Work out the finished part from the listing and answer in its coordinate system (mm). A direction names the side the tool comes from. Coordinates: 2 decimals unless noted, no trailing zeros. Order: outer loops, then holes, each group sorted by start corner. A loop starts at its lowest first (then second) coordinate and runs counter-clockwise, first axis right, second up.
1. The part is cut by section C-C, the plane y = -0.75. Give the vertices of the cut face in (x, z).
2. The part is cut by section D-D, the plane x = 0.4. Give the vertices of the cut face in (y, z).
3. Find the intervals of material crossed by probe 1 along Z at (x, y) = (-1.3, -0.75); probe 2 along Y at (x, z) = (-1.25, -0.85); probe 3 along Z at (x, y) = (-0.75, 4), in increasing order.
4. The part is cut by section B-B, the plane z = 0. Give the vertices of the cut face in (x, y) (3 decimals).
5. The part is cut by section A-A, the plane x = 0. Give the vertices of the cut face in (y, z) (3 decimals), then the cut area to 3 significant figures.
6. A tool of negligible diameter and unlimited length cuts with its end or side. For faces 1 (the cylindrical face through (0.066, 0.493, 1.924)), 2 (the cylindrical face through (1.402, 2.405, 0.442)), from which of +Z, -Z, +X, -X, +Y, -Y can it reach the whole face along a straight path? Write none if from no direction.
7. Flat-ended cylindrical pins translate along their axes: pin 1 Ø1 at (x, y) = (-1, 2.5) entering from +Z; pin 2 Ø1.5 at (x, z) = (-0.5, 1) entering from -Y; pin 3 Ø1 at (y, z) = (-1.5, -0.5) entering from -X. Find the tip coordinate at first contact, or state that the pin passes through.
Autodesk Inventor part; units mm, degrees
ref_plane "YZ Plane" through (0, 0, 0) normal (1, 0, 0) x (0, 1, 0)
ref_plane "XZ Plane" through (0, 0, 0) normal (0, 1, 0) x (-1, 0, 0)
ref_plane "XY Plane" through (0, 0, 0) normal (0, 0, 1) x (1, 0, 0)
sketch "Sketch1" plane through (0, 0, 0) normal (0, 1, 0) x (-1, 0, 0)
  arc A0 (1.2065, -1.5) -> (-1.2065, -1.5) centre (0, 0) ccw
  circle A1 centre (0, 0) radius 1.5
  line L0 (0, -1.5) -> (1.2065, -1.5)
  line L1 (0, -1.5) -> (-1.2065, -1.5)
  dimension "d1" = 3
  dimension "d0" = 3.85
extrude "Extrusion1" add sketch "Sketch1" along normal blind 1 contours A1 | L0 L1 A0
sketch "Sketch2" plane through (0, 1, 0) normal (0, 1, 0) x (1, 0, 0)
  arc A0 (-1.2065, 1.5) -> (1.2065, 1.5) centre (0, 0) ccw
  circle A1 centre (0, 0) radius 1.47
  dimension "d4" = 2.94
extrude "Extrusion2" add sketch "Sketch2" along normal blind 4.32
fillet "Fillet1" radius 1.47 1 edges at (-1.47, 5.32, 0)
sketch "Sketch3" plane through (0, 0, 0) normal (0, -1, 0) x (1, 0, 0)
  circle A0 centre (1.27, 0) radius 0.25
  circle A1 centre (-1.27, 0) radius 0.25
  point P0 (0, 0)
  dimension "d8" = 0.5
  dimension "d9" = 0.5
  dimension "d10" = 1.27
  dimension "d11" = 1.27
extrude "Extrusion3" add sketch "Sketch3" along normal blind 4.32
properties part number "3mm_LED"
Geometry says:
1. outline: circle Ø0.5 at (-1.27, 0); circle Ø0.5 at (1.27, 0)
2. outline: (0, -1.5) - (1, -1.5) - (1, -1.41) - (3.85, -1.41) arc R1.41 ccw to (3.85, 1.41) - (1, 1.41) - (1, 1.88) - (0, 1.88) - close
3. probe 1: z = -0.25 to 0.25
3. probe 2: y = 0 to 1
3. probe 3: z = -1.26 to 1.26
4. outline: (-1.925, 0) - (-1.52, 0) - (-1.52, -4.32) - (-1.02, -4.32) - (-1.02, 0) - (1.02, 0) - (1.02, -4.32) - (1.52, -4.32) - (1.52, 0) - (1.925, 0) - (1.925, 1) - (1.47, 1) - (1.47, 3.85) arc R1.47 ccw to (-1.47, 3.85) - (-1.47, 1) - (-1.925, 1) - close
5. outline: (0, -1.5) - (1, -1.5) - (1, -1.47) - (3.85, -1.47) arc R1.47 ccw to (3.85, 1.47) - (1, 1.47) - (1, 1.925) - (0, 1.925) - close
5. area: 15.2 mm2
6. face 1: +Y, -Y
6. face 2: +Y
7. pin 1: stops at z = 1.38
7. pin 2: stops at y = 0
7. pin 3: stops at x = -1.52
